```python
from build123d import *

# Parameters (mm, degrees)
SKETCH1_W           = 80
SKETCH1_H           = 50
BOSS_EXTRUDE1_DEPTH = 3
CUT_EXTRUDE1_REACH  = 49.265
SKETCH2_R           = 3
SKETCH3_W           = 3
SKETCH3_H           = 50
BOSS_EXTRUDE2_DEPTH = 30
FILLET1_RADIUS      = 25
FILLET1_LENGTH      = 3
FILLET2_RADIUS      = 25
FILLET2_LENGTH      = 3
SKETCH4_R           = 2.5
CUT_EXTRUDE2_DEPTH  = 200


with BuildPart() as part:
    # Sketch1 → Boss-Extrude1 (new body)
    with BuildSketch(Plane.XY):
        Rectangle(SKETCH1_W, SKETCH1_H)
    extrude(amount=BOSS_EXTRUDE1_DEPTH)

    # Sketch2 → Cut-Extrude1 (cut, up to next)
    with BuildSketch(Plane(origin=(0, 0, 0), x_dir=(-1, 0, 0), z_dir=(0, 0, -1)), mode=Mode.PRIVATE) as cut_extrude1_sk1:
        with Locations((-30, 0)):
            Circle(SKETCH2_R)
    cut_extrude1_tool1 = extrude(cut_extrude1_sk1.sketch, amount=-CUT_EXTRUDE1_REACH, mode=Mode.PRIVATE) & part.part
    # Sketch2 → Cut-Extrude1 (cut, up to next)
    with BuildSketch(Plane(origin=(0, 0, 0), x_dir=(-1, 0, 0), z_dir=(0, 0, -1)), mode=Mode.PRIVATE) as cut_extrude1_sk2:
        with Locations((30, 0)):
            Circle(SKETCH2_R)
    cut_extrude1_tool2 = extrude(cut_extrude1_sk2.sketch, amount=-CUT_EXTRUDE1_REACH, mode=Mode.PRIVATE) & part.part
    add(cut_extrude1_tool1.solids().sort_by_distance((30, 0, 0))[0], mode=Mode.SUBTRACT)
    add(cut_extrude1_tool2.solids().sort_by_distance((-30, 0, 0))[0], mode=Mode.SUBTRACT)

    # Sketch3 → Boss-Extrude2 (add)
    with BuildSketch(Plane(origin=(0, 0, 0), x_dir=(-1, 0, 0), z_dir=(0, 0, -1))):
        with Locations((-38.5, 0)):
            Rectangle(SKETCH3_W, SKETCH3_H)
        with Locations((38.5, 0)):
            Rectangle(SKETCH3_W, SKETCH3_H)
    extrude(amount=BOSS_EXTRUDE2_DEPTH)

    # Fillet1: full round fillet: the end face becomes a half cylinder, R = half its width
    fillet1_face = Plane((38.5, 0, -30), x_dir=(-1, 0, 0), z_dir=(0, 0, -1))  # on the end face: x along it, z out of the body
    fillet1_slab = fillet1_face.offset(-FILLET1_RADIUS / 2) * Box(FILLET1_LENGTH, 2 * FILLET1_RADIUS, FILLET1_RADIUS, mode=Mode.PRIVATE)  # the body's end, R deep
    fillet1_round = Plane((38.5, 0, -5), x_dir=(0, 0, -1), z_dir=(-1, 0, 0)) * Cylinder(FILLET1_RADIUS, FILLET1_LENGTH, mode=Mode.PRIVATE)  # its axis R under the face
    add(fillet1_slab - fillet1_round, mode=Mode.SUBTRACT)

    # Fillet2: full round fillet: the end face becomes a half cylinder, R = half its width
    fillet2_face = Plane((-38.5, 0, -30), x_dir=(1, 0, 0), z_dir=(0, 0, -1))  # on the end face: x along it, z out of the body
    fillet2_slab = fillet2_face.offset(-FILLET2_RADIUS / 2) * Box(FILLET2_LENGTH, 2 * FILLET2_RADIUS, FILLET2_RADIUS, mode=Mode.PRIVATE)  # the body's end, R deep
    fillet2_round = Plane((-38.5, 0, -5), x_dir=(0, 0, -1), z_dir=(1, 0, 0)) * Cylinder(FILLET2_RADIUS, FILLET2_LENGTH, mode=Mode.PRIVATE)  # its axis R under the face
    add(fillet2_slab - fillet2_round, mode=Mode.SUBTRACT)

    # Sketch4 → Cut-Extrude2 (cut)
    with BuildSketch(Plane(origin=(40, 0, 0), x_dir=(0, 0, -1), z_dir=(1, 0, 0))):
        with Locations((22, 0)):
            Circle(SKETCH4_R)
    extrude(amount=-CUT_EXTRUDE2_DEPTH, mode=Mode.SUBTRACT)


solid = part.part
```
Can you work these out from the model? Positions are in its coordinate system, mm. A direction names the side the tool comes from. Round coordinates to 2 decimals unless told otherwise and drop trailing zeros. Loops run counter-clockwise (first coordinate to the right, second up) from the corner with the lowest first, then second, coordinate; pieces in that order, holes last. Notation, with made-up numbers: M 60.5,-24 L 77.5,-24 A19 cw 77.5,6 Z; hole C 15,17 d7. An arc over 180 degrees is marked long. Answer as a JSON object with one key per item and string values. Group by question number.
Q1. Imagine slicing it at A-A, the plane z = -2.5. Please give me the cut outline in (x, y), then the cut area to 3 significant figures.
Q2. Imagine slicing it at B-B, the plane x = -30. Please give me the cut outline in (y, z), then the cut area to 3 significant figures.
Q3. We'd pull the mould along Y, two halves only. Please class faces 1 (the flat face through (-1, 0, 3)), 2 (the flat face through (0, 25, 1)), 3 (the cylindrical face through (-38.5, 0.1, -19.5)), 4 (the cylindrical face through (-38.479, -0.55, -29.994)): +Y half, -Y half, draft (parallel to the pull), parting line (faces both ways), or undercut.
Q4. Will these pins go through, and if not, where does the flat tip stop? pin 1 (6.5 mm diameter, centred on y = 0, z = -22, fed in from -X); pin 2 (12 mm diameter, centred on x = -24, y = -10, fed in from -Z).
Q5. Imagine slicing it at D-D, the plane z = -22. Please give me the cut outline in (x, y).
Q6. Imagine slicing it at C-C, the plane y = 0. Please give me the cut outline in (x, z), then the cut area to 3 significant figures.
Q7. On a 3-axis mill with a long thin cutter (end or side, diameter ignored), from which of +Z, -Z, +X, -X, +Y, -Y can I reach the whole of each face in a straight line? I mean faces 5 (the flat face through (37, 0, -11)), 6 (the cylindrical face through (-27, 0, 1)). Say none if no direction works.
Q8. Please list where these lines run through material, in increasing order: L1, parallel to Y at x = -30, z = 1.35; L2, parallel to X at y = 0.5, z = -11; L3, parallel to Z at x = 1, y = -1.5.
Findings:
{
 "1": {"outline": "M -40,-25 L -37,-25 L -37,25 L -40,25 Z; M 37,-25 L 40,-25 L 40,25 L 37,25 Z", "area": "300 mm2"},
 "2": {"outline": "M -25,0 L -3,0 L -3,3 L -25,3 Z; M 3,0 L 25,0 L 25,3 L 3,3 Z", "area": "132 mm2"},
 "3": {"face 1": "draft", "face 2": "+Y half", "face 3": "undercut", "face 4": "parting line"},
 "4": {"pin 1": "stops at x = -40", "pin 2": "stops at z = 0"},
 "5": {"outline": "M -40,-18.33 L -37,-18.33 L -37,-2.5 L -40,-2.5 Z; M -40,2.5 L -37,2.5 L -37,18.33 L -40,18.33 Z; M 37,-18.33 L 40,-18.33 L 40,-2.5 L 37,-2.5 Z; M 37,2.5 L 40,2.5 L 40,18.33 L 37,18.33 Z"},
 "6": {"outline": "M -40,-30 L -37,-30 L -37,-24.5 L -40,-24.5 Z; M -40,-19.5 L -37,-19.5 L -37,0 L -33,0 L -33,3 L -40,3 Z; M -27,0 L 27,0 L 27,3 L -27,3 Z; M 33,0 L 37,0 L 37,-19.5 L 40,-19.5 L 40,3 L 33,3 Z; M 37,-30 L 40,-30 L 40,-24.5 L 37,-24.5 Z", "area": "354 mm2"},
 "7": {"face 5": "-Z, +Y, -Y", "face 6": "+Z, -Z"},
 "8": {"L1": "y = -25 to -3, 3 to 25", "L2": "x = -40 to -37, 37 to 40", "L3": "z = 0 to 3"}
}
